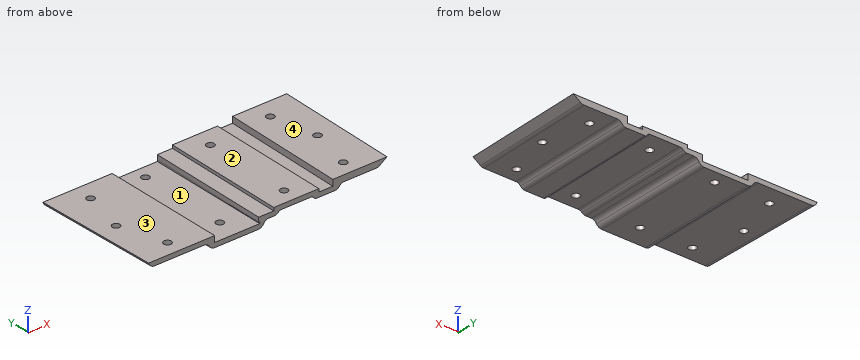
Autodesk Inventor part; units mm, degrees
ref_plane "Work Plane1" through (0, -41.25, 0) normal (0, 1, 0) x (-1, 0, 0)
ref_plane "YZ Plane" through (0, 0, 0) normal (1, 0, 0) x (0, 1, 0)
ref_plane "XY Plane" through (0, 0, 0) normal (0, 0, 1) x (1, 0, 0)
sketch "Sketch1" plane through (0, 0, 0) normal (0, 0, 1) x (1, 0, 0)
  line L0 (0, 0) -> (81, 0)
  line L1 (0, 0) -> (0, -41.25)
  line L2 (0, -41.25) -> (76.5595, -41.25)
  line L3 (10.5, 0) -> (10.5, -41.25)
  line L4 (30.5, 0) -> (29.4198, -41.25)
  line L5 (30.5, 0) -> (71.7641, 0) construction
  line L6 (50.5, 0) -> (49.0595, -41.25)
  line L7 (70.5, 0) -> (68.699, -41.25)
  line L8 (78, 0) -> (76.5595, -41.25)
  line L9 (78, 0) -> (119.2751, 0) construction
  line L10 (76.5595, -41.25) -> (81, 0)
  line L11 (3, 0) -> (3, -41.25)
  line L12 (18, 0) -> (18, -41.25)
  line L13 (23, 0) -> (21.9198, -41.25)
  line L14 (23, 0) -> (64.2641, 0) construction
  line L15 (38, 0) -> (36.9198, -41.25)
  line L16 (38, 0) -> (79.2641, 0) construction
  line L17 (43, 0) -> (41.5595, -41.25)
  line L18 (43, 0) -> (84.2751, 0) construction
  line L19 (58, 0) -> (56.5595, -41.25)
  line L20 (58, 0) -> (99.2751, 0) construction
  line L21 (63, 0) -> (61.199, -41.25)
  line L22 (63, 0) -> (104.2893, 0) construction
  line L23 (29.4198, -41.25) -> (29.6031, -34.2524)
  line L24 (29.6031, -34.2524) -> (30.3884, -4.2627)
  line L25 (49.0595, -41.25) -> (49.234, -36.253)
  line L26 (49.234, -36.253) -> (50.281, -6.2713)
  line L27 (68.699, -41.25) -> (68.9171, -36.2548)
  line L28 (68.9171, -36.2548) -> (70.2257, -6.2833)
  circle A0 centre (10.5, -6.25) radius 1.25
  circle A1 centre (10.5, -36.25) radius 1.25
  circle A2 centre (30.3884, -4.2627) radius 1.25
  circle A3 centre (29.6031, -34.2524) radius 1.25
  circle A4 centre (50.281, -6.2713) radius 1.25
  circle A5 centre (49.234, -36.253) radius 1.25
  circle A6 centre (70.2257, -6.2833) radius 1.25
  circle A7 centre (68.9171, -36.2548) radius 1.25
  line L29 (10.5, -6.25) -> (10.5, -21.25)
  line L30 (10.5, -21.25) -> (6.218, -21.25)
  circle A8 centre (6.218, -21.25) radius 1.25
  line L31 (6.218, -21.25) -> (73.0178, -21.4249)
  line L32 (6.218, -21.25) -> (73.018, -21.25) construction
  circle A9 centre (73.0178, -21.4249) radius 1.25
  dimension "d10" = 92
  dimension "d11" = 91.5
  dimension "d12" = 91.5
  dimension "d13" = 92
  dimension "d14" = 92
  dimension "d15" = 92.5
  dimension "d67" = 2.5
  dimension "d68" = 2.5
  dimension "d69" = 2.5
  dimension "d70" = 2.5
  dimension "d71" = 2.5
  dimension "d72" = 2.5
  dimension "d73" = 2.5
  dimension "d74" = 2.5
  dimension "d77" = 15
  dimension "d78" = 4.282
  dimension "d79" = 2.5
  dimension "d80" = 66.8
  dimension "d81" = 0.15
  dimension "d82" = 2.5
sketch "Sketch2" plane through (0, 0, 0) normal (0, 1, 0) x (-1, 0, 0)
  line L0 (-43, 0) -> (-58, 0)
  line L1 (-58, 0) -> (-58, 1)
  line L2 (-58, 1) -> (-43, 1)
  line L3 (-43, 1) -> (-43, 0)
  line L4 (-64.4672, 0) -> (-78, 0)
  line L5 (-78, 0) -> (-78, 2)
  line L6 (-78, 2) -> (-63, 2)
  line L7 (-63, 2) -> (-63, 0)
  line L8 (-23, 0) -> (-21.9198, 0)
  line L9 (-30.5, 0) -> (-29.4198, 0)
  line L10 (-23, 0) -> (-38, 0)
  line L11 (-38, 0) -> (-38, -2)
  line L12 (-38, -2) -> (-23, -2)
  line L13 (-23, -2) -> (-23, 0)
  line L14 (0, 0) -> (-23, 0)
  line L15 (-23, 0) -> (-23, -1.5)
  line L16 (-21.5, -1.5) -> (0, -1.5)
  line L17 (0, -1.5) -> (0, 0)
  line L18 (-23, 0) -> (-21.5, 0)
  line L19 (-21.5, -1.5) -> (-21.5, -3.5)
  line L20 (-21.5, -3.5) -> (-23, -3.5)
  line L21 (-23, -2) -> (-23, 0)
  line L22 (-23, -2) -> (-38, -2)
  line L23 (-39.5, -2) -> (-39.5, -3.5)
  line L24 (-39.5, -3.5) -> (-23, -3.5)
  line L25 (-39.5, -2) -> (-39.5, -1.5)
  line L26 (-39.5, 0) -> (-38, 0)
  line L27 (-38, 0) -> (-38, -2)
  line L28 (-38, 0) -> (-43, 0)
  line L29 (-43, -0.5) -> (-43, -1.5)
  line L30 (-43, -1.5) -> (-39.5, -1.5)
  line L31 (-38, -1.5) -> (-38, 0)
  line L32 (-43, 1) -> (-58, 1)
  line L33 (-58, 1) -> (-58, 0)
  line L34 (-56.5, -0.5) -> (-44, -0.5)
  line L35 (-43, -0.5) -> (-43, 1)
  line L36 (-38, 0) -> (-44, 0)
  line L37 (-44, -0.5) -> (-44, -1.5)
  line L38 (-44, -1.5) -> (-38, -1.5)
  line L39 (-38, -1.5) -> (-38, 0)
  line L40 (-56.5, 0) -> (-63, 0)
  line L41 (-64.4672, 0) -> (-64.4672, -1.5)
  line L42 (-64.4672, -1.5) -> (-56.5, -1.5)
  line L43 (-56.5, -1.5) -> (-56.5, -0.5)
  line L44 (-81, 2) -> (-78, 2)
  line L45 (-81, 2) -> (-78, 0)
  line L46 (-18, 0) -> (-18, -1.5)
  line L47 (0, 0) -> (-18, 0)
  line L48 (-18, 0) -> (-18, -1.5)
  line L49 (-18, -1.5) -> (0, -1.5)
  line L50 (0, -1.5) -> (0, 0)
  line L51 (-18, -1.5) -> (-18, 0)
  line L52 (-23, 0) -> (-23, -2)
  line L53 (-38, -2) -> (-38, 0)
  line L54 (-43, 0) -> (-43, -1.5)
  line L55 (-18, -1.5) -> (-21.5, -1.5)
  line L56 (-38, -2) -> (-23, -2)
  line L57 (-23, -2) -> (-23, 0)
  line L58 (-23, 0) -> (-18, 0)
  line L59 (-18, 0) -> (-18, -1.5)
  line L60 (-18, 0) -> (-23, 0)
  line L61 (-23, 0) -> (-23, -1.5)
  line L62 (-23, -1.5) -> (-18, -1.5)
  line L63 (-18, -1.5) -> (-18, 0)
  line L64 (-23, 0) -> (-21.5, 0)
  line L65 (-21.5, 0) -> (-21.5, -3.5)
  line L66 (-21.5, -3.5) -> (-23, -3.5)
  line L67 (-23, -3.5) -> (-23, 0)
  line L68 (-21.5, -3.5) -> (-39.5, -3.5)
  line L69 (-39.5, -3.5) -> (-39.5, -2)
  line L70 (-39.5, -2) -> (-21.5, -2)
  line L71 (-21.5, -2) -> (-21.5, -3.5)
  line L72 (-39.5, -2) -> (-38, -2)
  line L73 (-38, -2) -> (-38, 0)
  line L74 (-38, 0) -> (-39.5, 0)
  line L75 (-39.5, 0) -> (-39.5, -2)
  line L76 (-38, 0) -> (-44, 0)
  line L77 (-44, 0) -> (-44, -1.5)
  line L78 (-44, -1.5) -> (-38, -1.5)
  line L79 (-38, -1.5) -> (-38, 0)
  line L80 (-44, -0.5) -> (-58, -0.5)
  line L81 (-58, -0.5) -> (-58, 1)
  line L82 (-58, 1) -> (-44, 1)
  line L83 (-44, 1) -> (-44, -0.5)
  line L84 (-58, 1) -> (-56.5, 1)
  line L85 (-56.5, 1) -> (-56.5, -1.5)
  line L86 (-56.5, -1.5) -> (-58, -1.5)
  line L87 (-58, -1.5) -> (-58, 1)
  line L88 (-56.5, -1.5) -> (-64.4672, -1.5)
  line L89 (-64.4672, -1.5) -> (-64.4672, 0)
  line L90 (-64.4672, 0) -> (-56.5, 0)
  line L91 (-56.5, 0) -> (-56.5, -1.5)
  line L92 (-63, 0) -> (-78, 0)
  line L93 (-78, 0) -> (-78, 2)
  line L94 (-78, 2) -> (-63, 2)
  line L95 (-63, 2) -> (-63, 0)
  point P0 (-50.5, 0)
  point P1 (-58, 0)
  point P2 (-70.5, 0)
  point P3 (-81, 0)
  dimension "d24" = 1.5
  dimension "d29" = 6
ref_plane "Work Plane1" through (0, -41.25, 0) normal (0, 1, 0) x (-1, 0, 0)
sketch "Sketch3" plane through (0, -41.25, 0) normal (0, 1, 0) x (-1, 0, 0)
  line L0 (-23, 0) -> (-21.9198, 0)
  line L1 (-30.5, 0) -> (-29.4198, 0)
  line L2 (-38, 0) -> (-36.9198, 0)
  line L3 (-43, 0) -> (-41.5595, 0)
  line L4 (-50.5, 0) -> (-49.0595, 0)
  line L5 (-58, 0) -> (-56.5595, 0)
  line L6 (-63, 0) -> (-61.199, 0)
  line L7 (-70.5, 0) -> (-68.699, 0)
  line L8 (-78, 0) -> (-76.5595, 0)
  point P0 (0, 0)
  point P1 (-3, 0)
  point P2 (-3, 0)
  point P3 (-3, 0)
  point P4 (-10.5, 0)
  point P5 (-10.5, 0)
  point P6 (-10.5, 0)
  point P7 (-18, 0)
  point P8 (-18, 0)
  point P9 (-18, 0)
sketch "Sketch4" plane through (0, -41.25, 0) normal (0, 1, 0) x (-1, 0, 0)
  line L0 (0, 0) -> (-76.5595, 0)
  line L1 (-23, 0) -> (-21.9198, 0)
  line L2 (-30.5, 0) -> (-29.4198, 0)
  line L3 (-38, 0) -> (-36.9198, 0)
  line L4 (-43, 0) -> (-41.5595, 0)
  line L5 (-50.5, 0) -> (-49.0595, 0)
  line L6 (-58, 0) -> (-56.5595, 0)
  line L7 (-63, 0) -> (-61.199, 0)
  line L8 (-70.5, 0) -> (-68.699, 0)
  line L9 (-78, 0) -> (-76.5595, 0)
  line L10 (-21.9198, 0) -> (-36.9198, 0)
  line L11 (-36.9198, 0) -> (-36.9198, -2)
  line L12 (-36.9198, -2) -> (-21.9198, -2)
  line L13 (-21.9198, -2) -> (-21.9198, 0)
  line L14 (-41.5595, 0) -> (-56.5595, 0)
  line L15 (-56.5595, 0) -> (-56.5595, 1)
  line L16 (-56.5595, 1) -> (-41.5595, 1)
  line L17 (-41.5595, 1) -> (-41.5595, 0)
  line L18 (-61.199, 0) -> (-76.199, 0)
  line L19 (-76.199, 0) -> (-76.199, 2)
  line L20 (-76.199, 2) -> (-61.199, 2)
  line L21 (-61.199, 2) -> (-61.199, 0)
  point P0 (-3, 0)
  point P1 (-3, 0)
  point P2 (-3, 0)
  point P3 (-10.5, 0)
  point P4 (-10.5, 0)
  point P5 (-10.5, 0)
  point P6 (-18, 0)
  point P7 (-18, 0)
  point P8 (-18, 0)
  point P9 (-3, 0)
  point P10 (-10.5, 0)
  point P11 (-18, 0)
  dimension "d17" = 15
  dimension "d18" = 2
  dimension "d19" = 1
  dimension "d20" = 15
  dimension "d21" = 2
sketch "Sketch5" plane through (0, 0, 0) normal (0, 1, 0) x (-1, 0, 0)
  point P0 (0, 0)
sweep "Sweep1" add profiles "Sketch2" path "Sketch1" path curves L3 contours L14 L17 L16 L46
sweep "Sweep2" add profiles "Sketch2" path "Sketch1" path curves L13 contours L8 L14 L65 L62 L13 | L14 L46 L16 L65
sweep "Sweep3" add profiles "Sketch2" path "Sketch1" path curves L4 contours L70 L12 L67 L24 L23 | L70 L19 L20 L67
sweep "Sweep4" add profiles "Sketch2" path "Sketch1" path curves L4 contours L70 L19 L20 L67 | L13 L62 L19 L70
sketch3d "3D Sketch1"
  line L0 (39.5, 0, -2) -> (38.4198, -41.25, -2)
sweep "Sweep5" add profiles "Sketch2" path "3D Sketch1" contours L26 L11 L38 L75 | L38 L11 L70 L25
sweep "Sweep6" add profiles "Sketch2" path "Sketch1" path curves L17 contours L35 L29 L38 L37 L77 L0 | L28 L75 L30 L29 L35 | L26 L11 L38 L75
sweep "Sweep7" add profiles "Sketch2" path "Sketch1" path curves L6 contours L0 L83 L2 L3 | L0 L85 L2 L83 | L0 L1 L2 L85
sweep "Sweep8" add profiles "Sketch2" path "Sketch1" path curves L6 contours L77 L34 L85 L0 | L0 L85 L2 L83 | L85 L80 L81 L0 | L0 L1 L2 L85
sweep "Sweep9" add profiles "Sketch2" path "Sketch1" path curves L19 contours L85 L80 L81 L0 | L0 L1 L2 L85 | L43 L42 L87 L80
sketch3d "3D Sketch2"
  line L0 (58, 0, 1) -> (56.5595, -41.25, 1)
sweep "Sweep10" add profiles "Sketch2" path "3D Sketch2" contours L85 L80 L81 L0 | L81 L87 L42 L41 L90 L40 | L43 L42 L87 L80
sweep "Sweep11" add profiles "Sketch2" path "Sketch1" path curves L21 contours L90 L4 L5 L6 L7
sketch3d "3D Sketch3"
  line L0 (78, 0, 2) -> (76.199, -41.25, 2)
sweep "Sweep12" add profiles "Sketch2" path "3D Sketch3" contours L5 L45 L44
fillet "Fillet1" radius 2 1 edges at (77.0995, -20.625, 0)
fillet "Fillet2" radius 2 2 edges at (63.7469, -20.625, -1.5) (63.7469, -20.625, 0)
fillet "Fillet3" radius 1 2 edges at (55.7798, -20.625, -1.5) (55.7798, -20.625, -0.5)
fillet "Fillet4" radius 2 2 edges at (43.2798, -20.625, -0.5) (43.2798, -20.625, -1.5)
fillet "Fillet5" radius 2 2 edges at (38.9599, -20.625, -1.5) (38.9599, -20.625, -3.5)
fillet "Fillet6" radius 2 2 edges at (20.9599, -20.625, -3.5) (20.9599, -20.625, -1.5)
fillet "Fillet7" radius 2 1 edges at (0, -20.625, -1.5)
extrude "Extrusion1" cut sketch "Sketch1" along normal through all both and the other way through all contours A0 L3 | L3 A0 | A1 L3 | L3 A1 | A2 L4 | L4 A2 | A3 L4 | L4 A3 | A4 L6 | L6 A4 | A5 L6 | L6 A5 | A6 L7 | L7 A6 | A7 L7 | L7 A7
extrude "Extrusion2" cut sketch "Sketch1" along normal through all both and the other way through all contours L31 L30 A8 | A8 L30 L31 | A9
properties part number "Finger_Screwing_Cage_1"
The listing builds one solid part. Answer for the finished solid, in the listing's coordinates (mm). Face numbers are marked on the shaded views. A direction names the side the tool comes from. Round coordinates to 2 decimals unless told otherwise and drop trailing zeros. Answer as CSV lines item,"result". Start each with the question number.
(1) Find the intervals of material crossed by probe 1 along X at (y, z) = (-37, -1.3); probe 2 along Z at (x, y) = (36.5, -25); probe 3 along Z at (x, y) = (10.5, -1.5), in increasing order. Write a range as from..to.
(2) Flat-ended cylindrical pins translate along their axes: pin 1 Ø5 at (x, y) = (49.5, -22) entering from +Z; pin 2 Ø1.5 at (x, y) = (10.5, -6.25) entering from -Z; pin 3 Ø4 at (x, y) = (10.5, -36.25) entering from +Z; pin 4 Ø9 at (x, y) = (13, -23.5) entering from -Z. Find the tip coordinate at first contact, or state that the pin passes through.
(3) For a pull along X with two mould halves and no side action, classify the marked faces 1 and 2 as +X half, -X half, draft (parallel to the pull), parting line (faces both ways), or undercut.
(4) A tool of negligible diameter and unlimited length cuts with its end or side. For the marked faces 3 and 4, from which of +Z, -Z, +X, -X, +Y, -Y can it reach the whole face along a straight path? Write none if from no direction.
Evaluation:
1,probe 1,"1.06..9.5, 11.5..22.03, 36.71..42.67, 55.34..62.86"
1,probe 2,"-3.5..-2"
1,probe 3,"-1.5..0"
2,pin 1,"z = 1"
2,pin 2,"through"
2,pin 3,"z = 0"
2,pin 4,"z = -1.5"
3,face 1,"undercut"
3,face 2,"draft"
4,face 3,"+Z, -X, +Y, -Y"
4,face 4,"+Z, +X, -X, +Y, -Y"
